Autodesk Inventor part; units mm, degrees
ref_plane "YZ Plane" through (0, 0, 0) normal (1, 0, 0) x (0, 1, 0)
ref_plane "XZ Plane" through (0, 0, 0) normal (0, 1, 0) x (-1, 0, 0)
ref_plane "XY Plane" through (0, 0, 0) normal (0, 0, 1) x (1, 0, 0)
sketch "Szkic1" plane through (0, 0, 0) normal (0, 0, 1) x (1, 0, 0)
  line L0 (0, 53.1646) -> (0, 0)
  line L1 (0, 0) -> (98.9175, 0)
  line L2 (98.9175, 0) -> (98.9175, 1.2597)
  line L3 (98.9175, 1.2597) -> (101.455, 3.8466)
  line L4 (101.455, 3.8466) -> (101.455, 38.0126)
  line L5 (101.455, 38.0126) -> (98.9175, 40.5017)
  line L6 (98.9175, 40.5017) -> (98.9175, 50.7051)
  line L7 (98.9175, 50.7051) -> (96.4101, 53.1646)
  line L8 (96.4101, 53.1646) -> (0, 53.1646)
  line L9 (-10, 93.1646) -> (141.455, 93.1646)
  line L10 (141.455, 93.1646) -> (141.455, -17)
  line L11 (141.455, -17) -> (-10, -17)
  line L12 (-10, -17) -> (-10, 93.1646)
  line L13 (91.455, 93.1646) -> (91.455, 43.1646)
  line L14 (91.455, 43.1646) -> (141.455, 43.1646)
  point P0 (-10, 13.9306)
  point P1 (7.9866, -17)
  dimension "d0" = 101.455
  dimension "d1" = 53.1646
  dimension "d2" = 98.9175
  dimension "d21" = 98.9175
  dimension "d22" = 1.2597
  dimension "d23" = 10.2034
  dimension "d24" = 34.166
  dimension "d33" = 40
  dimension "d34" = 40
  dimension "d35" = 17
  dimension "d36" = 10
  dimension "d37" = 50
  dimension "d38" = 50
extrude "Wyciągnięcie proste1" add sketch "Szkic1" along normal blind 2.5 contours L8 L13 L14 L6 L5 L4 L3 L2 L1 L0 | L0 L1 L2 L3 L4 L5 L6 L14 L10 L11 L12 L9 L13 L8
sketch "Szkic2" plane through (0, 0, 2.5) normal (0, 0, 1) x (1, 0, 0)
  line L0 (-10, 93.1646) -> (-10, -17)
  line L1 (-10, -17) -> (141.455, -17)
  line L2 (141.455, -17) -> (141.455, 43.1646)
  line L3 (141.455, 43.1646) -> (91.455, 43.1646)
  line L4 (91.455, 43.1646) -> (91.455, 93.1646)
  line L5 (91.455, 93.1646) -> (-10, 93.1646)
  line L6 (10, 93.1646) -> (10, 73.1646)
  line L7 (10, 73.1646) -> (71.455, 73.1646)
  line L8 (71.455, 73.1646) -> (71.455, 93.1646)
  line L9 (91.455, 93.1646) -> (-10, 93.1646)
  line L10 (141.455, -17) -> (141.455, 43.1646)
  line L11 (141.455, 23.1646) -> (121.455, 23.1646)
  line L12 (121.455, 23.1646) -> (121.455, 3)
  line L13 (121.455, 3) -> (141.455, 3)
  circle A0 centre (45, 28.0823) radius 37.5
  point P0 (0, 0)
  point P1 (131.455, -7)
  point P2 (131.455, 33.1646)
  point P3 (81.455, 83.1646)
  point P4 (0, 83.1646)
  point P5 (9.25, 63.8323)
  point P6 (80.75, 63.8323)
  point P7 (80.75, -7.6677)
  point P8 (9.25, -7.6677)
  dimension "d42" = 20
  dimension "d43" = 20
  dimension "d44" = 20
  dimension "d45" = 20
  dimension "d46" = 20
  dimension "d47" = 20
  dimension "d78" = 10
  dimension "d79" = 10
  dimension "d80" = 10
  dimension "d81" = 10
  dimension "d82" = 10
  dimension "d83" = 10
  dimension "d84" = 10
  dimension "d85" = 10
  dimension "d121" = 75
  dimension "d122" = 35.75
  dimension "d123" = 35.75
  dimension "d124" = 35.75
  dimension "d125" = 35.75
  dimension "d126" = 35.75
  dimension "d127" = 35.75
  dimension "d128" = 35.75
  dimension "d129" = 35.75
  dimension "d139" = 45.0823
  dimension "d140" = 101.455
  dimension "d141" = 90.1646
  dimension "d142" = 55
fillet "Zaokrąglenie1" radius 5 4 edges at (-10, 93.1646, 1.25) (91.455, 93.1646, 1.25) (141.455, 43.1646, 1.25) (141.455, -17, 1.25)
hole "Otwór1" at (131.455, -7, 2.5) at (131.455, 33.1646, 2.5) at (81.455, 83.1646, 2.5) at (0, 83.1646, 2.5) direction (0, 0, -1) diameter 4 end through all
fillet "Zaokrąglenie2" radius 2 1 edges at (-10, -17, 1.25)
sketch "Szkic4" plane through (0, 0, 2.5) normal (0, 0, 1) x (1, 0, 0)
  arc A0 (-10, -15) -> (-8, -17) centre (-8, -15) ccw
  line L0 (-8, -17) -> (136.455, -17)
  arc A1 (136.455, -17) -> (141.455, -12) centre (136.455, -12) ccw
  line L1 (141.455, -12) -> (141.455, 38.1646)
  arc A2 (141.455, 38.1646) -> (136.455, 43.1646) centre (136.455, 38.1646) ccw
  line L2 (136.455, 43.1646) -> (91.455, 43.1646)
  line L3 (91.455, 43.1646) -> (91.455, 88.1646)
  arc A3 (91.455, 88.1646) -> (86.455, 93.1646) centre (86.455, 88.1646) ccw
  line L4 (86.455, 93.1646) -> (-5, 93.1646)
  arc A4 (-5, 93.1646) -> (-10, 88.1646) centre (-5, 88.1646) ccw
  line L5 (-10, 88.1646) -> (-10, -15)
  circle A5 centre (81.455, 83.1646) radius 2
  circle A6 centre (131.455, -7) radius 2
  circle A7 centre (131.455, 33.1646) radius 2
  circle A8 centre (0, 83.1646) radius 2
  point P0 (0, 0)
  point P1 (-5.5, 53.1646)
  point P2 (-5.5, -12.5)
  point P3 (101.455, -12.5)
  dimension "d106" = 40
  dimension "d107" = 4.5
  dimension "d108" = 4.5
  dimension "d109" = 4.5
  dimension "d110" = 4.5
hole "Otwór2" at (-5.5, 53.1646, 2.5) at (-5.5, -12.5, 2.5) at (101.455, -12.5, 2.5) direction (0, 0, -1) diameter 3 end through all
chamfer "Faza2" distance 30 angle 45 1 edges at (91.455, 43.1646, 1.25)
extrude "Wyciągnięcie proste4" cut sketch "Szkic2" against normal through all contours L5 L8 L7 L6 | L13 L12 L11 L2 | A0
hole "Otwór3" at (9.25, 63.8323, 2.5) at (80.75, 63.8323, 2.5) at (80.75, -7.6677, 2.5) at (9.25, -7.6677, 2.5) direction (0, 0, -1) diameter 4 end through all
fillet "Zaokrąglenie3" radius 10 4 edges at (71.455, 73.1646, 1.25) (10, 73.1646, 1.25) (121.455, 23.1646, 1.25) (121.455, 3, 1.25)
fillet "Zaokrąglenie3" radius 5 4 edges at (141.455, 23.1646, 1.25) (141.455, 3, 1.25) (71.455, 93.1646, 1.25) (10, 93.1646, 1.25)
sketch "Szkic7" plane through (0, 0, 2.5) normal (0, 0, 1) x (1, 0, 0)
  arc A0 (10, 88.1646) -> (5, 93.1646) centre (5, 88.1646) ccw
  line L0 (5, 93.1646) -> (-5, 93.1646)
  arc A1 (-5, 93.1646) -> (-10, 88.1646) centre (-5, 88.1646) ccw
  line L1 (-10, 88.1646) -> (-10, -15)
  arc A2 (-10, -15) -> (-8, -17) centre (-8, -15) ccw
  line L2 (-8, -17) -> (136.455, -17)
  arc A3 (136.455, -17) -> (141.455, -12) centre (136.455, -12) ccw
  line L3 (141.455, -12) -> (141.455, -2)
  arc A4 (141.455, -2) -> (136.455, 3) centre (136.455, -2) ccw
  line L4 (136.455, 3) -> (131.455, 3)
  arc A5 (121.455, 13) -> (131.455, 3) centre (131.455, 13) ccw
  line L5 (121.455, 13) -> (121.455, 13.1646)
  arc A6 (131.455, 23.1646) -> (121.455, 13.1646) centre (131.455, 13.1646) ccw
  line L6 (131.455, 23.1646) -> (136.455, 23.1646)
  arc A7 (136.455, 23.1646) -> (141.455, 28.1646) centre (136.455, 28.1646) ccw
  line L7 (141.455, 28.1646) -> (141.455, 38.1646)
  arc A8 (141.455, 38.1646) -> (136.455, 43.1646) centre (136.455, 38.1646) ccw
  line L8 (136.455, 43.1646) -> (121.455, 43.1646)
  line L9 (91.455, 73.1646) -> (121.455, 43.1646)
  line L10 (91.455, 73.1646) -> (91.455, 88.1646)
  arc A9 (91.455, 88.1646) -> (86.455, 93.1646) centre (86.455, 88.1646) ccw
  line L11 (86.455, 93.1646) -> (76.455, 93.1646)
  arc A10 (76.455, 93.1646) -> (71.455, 88.1646) centre (76.455, 88.1646) ccw
  line L12 (71.455, 88.1646) -> (71.455, 83.1646)
  arc A11 (61.455, 73.1646) -> (71.455, 83.1646) centre (61.455, 83.1646) ccw
  line L13 (61.455, 73.1646) -> (20, 73.1646)
  arc A12 (10, 83.1646) -> (20, 73.1646) centre (20, 83.1646) ccw
  line L14 (10, 83.1646) -> (10, 88.1646)
  circle A13 centre (80.75, -7.6677) radius 2
  circle A14 centre (9.25, 63.8323) radius 2
  circle A15 centre (80.75, 63.8323) radius 2
  circle A16 centre (9.25, -7.6677) radius 2
  circle A17 centre (45, 28.0823) radius 37.5
  circle A18 centre (-5.5, -12.5) radius 1.5
  circle A19 centre (-5.5, 53.1646) radius 1.5
  circle A20 centre (101.455, -12.5) radius 1.5
  circle A21 centre (0, 83.1646) radius 2
  circle A22 centre (131.455, 33.1646) radius 2
  circle A23 centre (131.455, -7) radius 2
  circle A24 centre (81.455, 83.1646) radius 2
  line L15 (-10, 72.6646) -> (-4.5, 72.6646)
  arc A25 (-5, 93.1646) -> (-10, 88.1646) centre (-5, 88.1646) ccw
  line L16 (-4.5, 72.6646) -> (-4.5, 93.1646)
  point P0 (0, 0)
  dimension "d145" = 5.5
  dimension "d147" = 20.5
extrude "Wyciągnięcie proste5" cut sketch "Szkic7" against normal through all contours L16 L15 L1 A1 L0
equation "\"d47\" = d46"
properties part number "3DP_PLA_Controller_Case_Top"
Geometry: final body of the model. Coordinates: model frame, mm. A direction names the side the tool comes from. Give positions to 0.01 mm unless a question says otherwise; leave off trailing zeros. Loops run counter-clockwise (first coordinate to the right, second up) from the corner with the lowest first, then second, coordinate; pieces in that order, holes last. Notation, with made-up numbers: M 43.25,-3.75 L 94.25,-3.75 A25 cw 94.25,27.25 Z; hole C 47.5,38 d3. An arc over 180 degrees is marked long. Put each result on its own line as item: value. Start each with the question number.
1) Access query for faces 1 (the cylindrical face through (124.462, 5.852, 1.232)), 2 (the cylindrical face through (13.007, 76.016, 1.232)), 3 (the cylindrical face through (9.16, 65.83, 1.23)). Directions: +Z, -Z, +X, -X, +Y, -Y. A direction counts if a zero-diameter tool reaches every point of the face in a straight line with its end or side. Return the directions, or none.
2) Pull-direction query (X, two-part tool) for faces 4 (the flat face through (81.5, 38.9, 0)), 5 (the cylindrical face through (90.03, 91.66, 1.27)), 6 (the cylindrical face through (131.367, 35.163, 1.232)), 7 (the cylindrical face through (68.6, 76.17, 1.23)); classes: pulls with the +X half, pulls with the -X half, needs draft (parallel to the pull), parting line crosses it, or undercut.
3) Cut plane A-A (x = 0). Output: boundary loops of the cut face in (y, z), then the cut area to 3 significant figures.
4) Cut plane D-D (x = 105.5). Output: boundary loops of the cut face in (y, z).
5) Cut plane C-C (z = 1). Give the number of separate pieces and of enclosed holes in the cut face, then the cut area to 3 significant figures.
6) Contact query for flat-ended pins moving along their axis: pin 1 (0.8 mm diameter, centred on y = 86.5, z = 1.5, fed in from -X); pin 2 (1.2 mm diameter, centred on x = 31, z = 1, fed in from +Y). Output: stop coordinate, or through.
7) Ray query, line 1 along Y through (x, z) = (-5.5, 0.8); line 2 along Y through (x, z) = (0, 0.7); line 3 along Y through (x, z) = (45, 2.35). Return the intervals inside material, ascending.
8) Cut plane B-B (y = 0). Output: boundary loops of the cut face in (x, z), then the cut area to 3 significant figures.
Verdict:
1. face 1: +Z, -Z, +X
1. face 2: +Z, -Z, +Y
1. face 3: +Z, -Z
2. face 4: needs draft
2. face 5: pulls with the +X half
2. face 6: undercut
2. face 7: undercut
3. outline: M -17,0 L 81.16,0 L 81.16,2.5 L -17,2.5 Z; M 85.16,0 L 93.16,0 L 93.16,2.5 L 85.16,2.5 Z
3. area: 265 mm2
4. outline: M -17,0 L 59.12,0 L 59.12,2.5 L -17,2.5 Z
5. separate pieces: 1
5. enclosed holes: 12
5. area: 8,400 mm2
6. pin 1: x = -4.5
6. pin 2: y = 73.16
7. line 1: -17 to -14, -11 to 51.66, 54.66 to 72.66
7. line 2: -17 to 81.16, 85.16 to 93.16
7. line 3: -17 to -9.42, 65.58 to 73.16
8. outline: M -10,0 L 20.15,0 L 20.15,2.5 L -10,2.5 Z; M 69.85,0 L 141.04,0 L 141.04,2.5 L 69.85,2.5 Z
8. area: 253 mm2
